For this review, take the finished solid that the model builds, in its own axes (mm). Face numbers are marked on the shaded views. A direction names the side the tool comes from. Coordinates: 2 decimals unless noted, no trailing zeros. Write each loop counter-clockwise with the first axis right and the second up, starting at its lowest first coordinate (ties: lowest second). Pieces come first, ordered by that corner, then holes.
1) We need section A-A on y = -64. Write out the cut boundary in (x, z).
2) Mouldability with a two-part tool opening along X and no side actions: class the marked faces 3, 4 and 5 as pulls with the +X half, pulls with the -X half, needs draft (parallel to the pull), parting line crosses it, or undercut.
3) For the marked faces 1 and 2, list the 3-axis set-ups (+Z, -Z, +X, -X, +Y, -Y) from which the entire face can be reached by the end or side of a thin tool; tool diameter is ignored.
4) To check wall thickness, follow line 1 along Y through (x, z) = (0.9, -15); line 2 along Y through (x, z) = (15, -28.65); line 3 along Z through (x, y) = (12, -28). State the ranges of each line that lie inside material, in increasing order.
5) We need section C-C on z = -15. Write out the cut boundary in (x, y).
6) We need section B-B on x = 15. Give the number of separate pieces and of enclosed holes in the cut face, then the cut area to 3 significant figures.
7) We need section D-D on x = 7.25. Write out the cut boundary in (y, z), then the cut area to 3 significant figures.
from build123d import *

# Parameters (mm, degrees)
EXTRUDE_1_DEPTH          = 70
SKETCH_3_R               = 3
SKETCH_3_R_2             = 2
CUT_EXTRUDE_1_DEPTH      = 82.853527719
CUT_EXTRUDE_2_DEPTH      = 82.853527719
CUT_EXTRUDE_2_DEPTH_BACK = 82.853527719
SKETCH_4_R               = 3.5


with BuildPart() as part:
    # 草图2 → 凸台-拉伸1 (new, symmetric)
    with BuildSketch(Plane(origin=(0, 0, 0), x_dir=(1, 0, 0), z_dir=(0, 1, 0))):
        with BuildLine():
            Line((4, 0), (26, 0))
            ThreePointArc((26, 0), (28.828427125, 1.171572875), (30, 4))
            Line((30, 4), (30, 26))
            ThreePointArc((30, 26), (28.828427125, 28.828427125), (26, 30))
            Line((26, 30), (4, 30))
            ThreePointArc((4, 30), (1.171572875, 28.828427125), (0, 26))
            Line((0, 26), (0, 4))
            ThreePointArc((0, 4), (1.171572875, 1.171572875), (4, 0))
        make_face()
        with BuildLine():
            Line((4, 2), (26, 2))
            ThreePointArc((26, 2), (27.414213562, 2.585786438), (28, 4))
            Line((28, 4), (28, 26))
            ThreePointArc((28, 26), (27.414213562, 27.414213562), (26, 28))
            Line((26, 28), (4, 28))
            ThreePointArc((4, 28), (2.585786438, 27.414213562), (2, 26))
            Line((2, 26), (2, 4))
            ThreePointArc((2, 4), (2.585786438, 2.585786438), (4, 2))
        make_face(mode=Mode.SUBTRACT)
    extrude(amount=EXTRUDE_1_DEPTH, both=True)

    # 草图3 → 切除-拉伸1 (cut, through all)
    with BuildSketch(Plane.XY):
        with Locations((15, -64)):
            Circle(SKETCH_3_R)
        with Locations((15, -9)):
            Circle(SKETCH_3_R)
        with Locations((15, 55)):
            Circle(SKETCH_3_R_2)
    extrude(amount=-CUT_EXTRUDE_1_DEPTH, mode=Mode.SUBTRACT)

    # 草图4 → 切除-拉伸2 (cut, two sides: drawn at the far end of the back side and taken through both)
    with BuildSketch(Plane(origin=(0, 0, 0), x_dir=(0, 0, -1), z_dir=(1, 0, 0)).offset(-CUT_EXTRUDE_2_DEPTH_BACK)):
        with Locations(Location((15, -50, 0), (0, 0, 180))):
            Circle(SKETCH_4_R)
        with Locations(Location((15, 30, 0), (0, 0, 180))):
            Circle(SKETCH_4_R)
    extrude(amount=CUT_EXTRUDE_2_DEPTH + CUT_EXTRUDE_2_DEPTH_BACK, mode=Mode.SUBTRACT)


solid = part.part
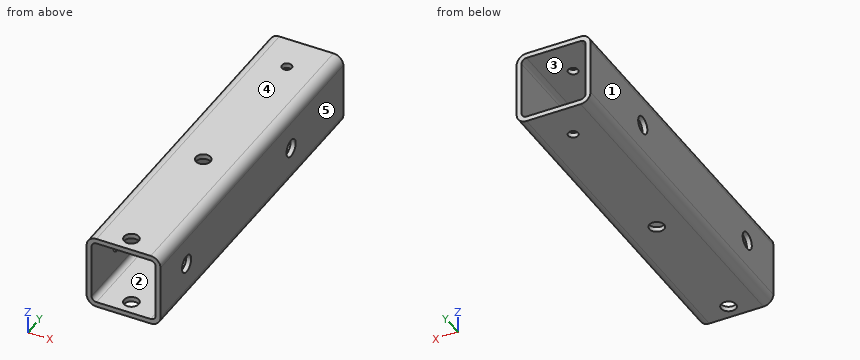
Result:
1. outline: (0, -26) arc R4 ccw to (4, -30) - (12, -30) - (12, -28) - (4, -28) arc R2 cw to (2, -26) - (2, -4) arc R2 cw to (4, -2) - (12, -2) - (12, 0) - (4, 0) arc R4 ccw to (0, -4) - close; (18, -30) - (26, -30) arc R4 ccw to (30, -26) - (30, -4) arc R4 ccw to (26, 0) - (18, 0) - (18, -2) - (26, -2) arc R2 cw to (28, -4) - (28, -26) arc R2 cw to (26, -28) - (18, -28) - close
2. face 3: undercut
2. face 4: needs draft
2. face 5: pulls with the +X half
3. face 1: +Z, -Z, -X, +Y, -Y
3. face 2: +Y, -Y
4. line 1: y = -70 to -53.5, -46.5 to 26.5, 33.5 to 70
4. line 2: y = -70 to -67, -61 to -12, -6 to 53, 57 to 70
4. line 3: z = -30 to -28, -2 to 0
5. outline: (0, -70) - (2, -70) - (2, -53.5) - (0, -53.5) - close; (0, -46.5) - (2, -46.5) - (2, 26.5) - (0, 26.5) - close; (0, 33.5) - (2, 33.5) - (2, 70) - (0, 70) - close; (28, -70) - (30, -70) - (30, -53.5) - (28, -53.5) - close; (28, -46.5) - (30, -46.5) - (30, 26.5) - (28, 26.5) - close; (28, 33.5) - (30, 33.5) - (30, 70) - (28, 70) - close
6. separate pieces: 8
6. enclosed holes: 0
6. area: 496 mm2
7. outline: (-70, -30) - (70, -30) - (70, -28) - (-70, -28) - close; (-70, -2) - (70, -2) - (70, 0) - (-70, 0) - close
7. area: 560 mm2
